Build history of the part. All positions in model axes, mm. Coordinates: 2 decimals unless noted, no trailing zeros. Loops run counter-clockwise (first coordinate to the right, second up) from the corner with the lowest first, then second, coordinate; pieces in that order, holes last. Notation, with made-up numbers: (-20, -30) - (32, -30) arc R11 cw to (32, -12) - close; hole circle Ø11 at (89.5, 36.25). An arc over 180 degrees is marked (long way). One line per item, written item: value.
Autodesk Inventor part; units mm, degrees
ref_plane "YZ Plane" through (0, 0, 0) normal (1, 0, 0) x (0, 1, 0)
ref_plane "XZ Plane" through (0, 0, 0) normal (0, 1, 0) x (-1, 0, 0)
ref_plane "XY Plane" through (0, 0, 0) normal (0, 0, 1) x (1, 0, 0)
sketch "スケッチ1" plane through (0, 0, 0) normal (0, 0, 1) x (1, 0, 0)
  line L0 (0, 0) -> (-15, 0) construction
  line L1 (0, 5) -> (-15, 5) construction
  line L2 (-15, -5) -> (0, -5) construction
  arc A0 (0, -5) -> (0, 5) centre (0, 0) ccw construction
  arc A1 (-15, 5) -> (-15, -5) centre (-15, 0) ccw
  circle A2 centre (-15, 0) radius 1.5
  circle A3 centre (0, 0) radius 1.5
  arc A4 (-0.65, 6.4674) -> (-0.65, -6.4674) centre (0, 0) ccw construction
  line L3 (-15.5, 4.9749) -> (-0.65, 6.4674)
  line L4 (-15.5, -4.9749) -> (-0.65, -6.4674)
  arc A5 (-0.65, -6.4674) -> (-0.65, 6.4674) centre (0, 0) ccw
  point P0 (-7.5, 0)
  dimension "d0" = 15
  dimension "d1" = 10
  dimension "d2" = 3
  dimension "d3" = 3
  dimension "d4" = 13
extrude "押し出し1" add sketch "スケッチ1" along normal blind 3
properties part number "ウィング抑え" material "ポリカーボネート、スモーク"
Item 1: Cut at A-A, the plane x = 0. Write the cut outline in (y, z), then the cut area to 3 significant figures.
Check result:
outline: (-6.5, 0) - (-1.5, 0) - (-1.5, 3) - (-6.5, 3) - close; (1.5, 0) - (6.5, 0) - (6.5, 3) - (1.5, 3) - close
area: 30.0 mm^2
Item 2: Cut at B-B, the plane z = 2.2. Write the cut outline in (x, y), then the cut area to 3 significant figures.
Check result:
outline: (-15.5, -4.97) - (-0.65, -6.47) arc R6.5 ccw (long way) to (-0.65, 6.47) - (-15.5, 4.97) arc R5 ccw to start; hole circle Ø3 at (-15, 0); hole circle Ø3 at (0, 0)
area: 265 mm^2
Item 3: Cut at D-D, the plane y = 3. Write the cut outline in (x, z), then the cut area to 3 significant figures.
Check result:
outline: (-19, 0) - (5.77, 0) - (5.77, 3) - (-19, 3) - close
area: 74.3 mm^2
Item 4: Cut at C-C, the plane x = -15. Write the cut outline in (y, z).
Check result:
outline: (-5.03, 0) - (-1.5, 0) - (-1.5, 3) - (-5.03, 3) - close; (1.5, 0) - (5.03, 0) - (5.03, 3) - (1.5, 3) - close
Item 5: Probe probe 1 along X at (y, z) = (-0.75, 1.2); probe 2 along X at (y, z) = (1, 0.8); probe 3 along Y at (x, z) = (0, 0.75). List the from-to ranges inside material, lowest first. Write a range as from..to.
Check result:
probe 1: x = -19.94..-16.3, -13.7..-1.3, 1.3..6.46
probe 2: x = -19.9..-16.12, -13.88..-1.12, 1.12..6.42
probe 3: y = -6.5..-1.5, 1.5..6.5
Item 6: Drop a flat-ended pin along its axis: P1, Ø1, axis at x = -15.5, z = 2.5, coming from the -Y side. Give the stop position or say it passes through.
Check result:
P1: stops at y = -5.03
Item 7: Pull direction Y, two halves, no side cores. Call faces 1 (the face through (-7, 0, 0)), 2 (the face through (-1.5, -0.07, 1.48)), 3 (the face through (-20, 0, 1)): released by +Y, released by -Y, zero draft, split by the parting line, or undercut.
Check result:
face 1: zero draft
face 2: undercut
face 3: split by the parting line
